Design review of the part shown in the three views and the two pictorial views. Dimensions are in mm from the part's minimum x, y and z. Give positions to 0.01 mm unless a question says otherwise; leave off trailing zeros. Loops run counter-clockwise (first coordinate to the right, second up) from the corner with the lowest first, then second, coordinate; pieces in that order, holes last.
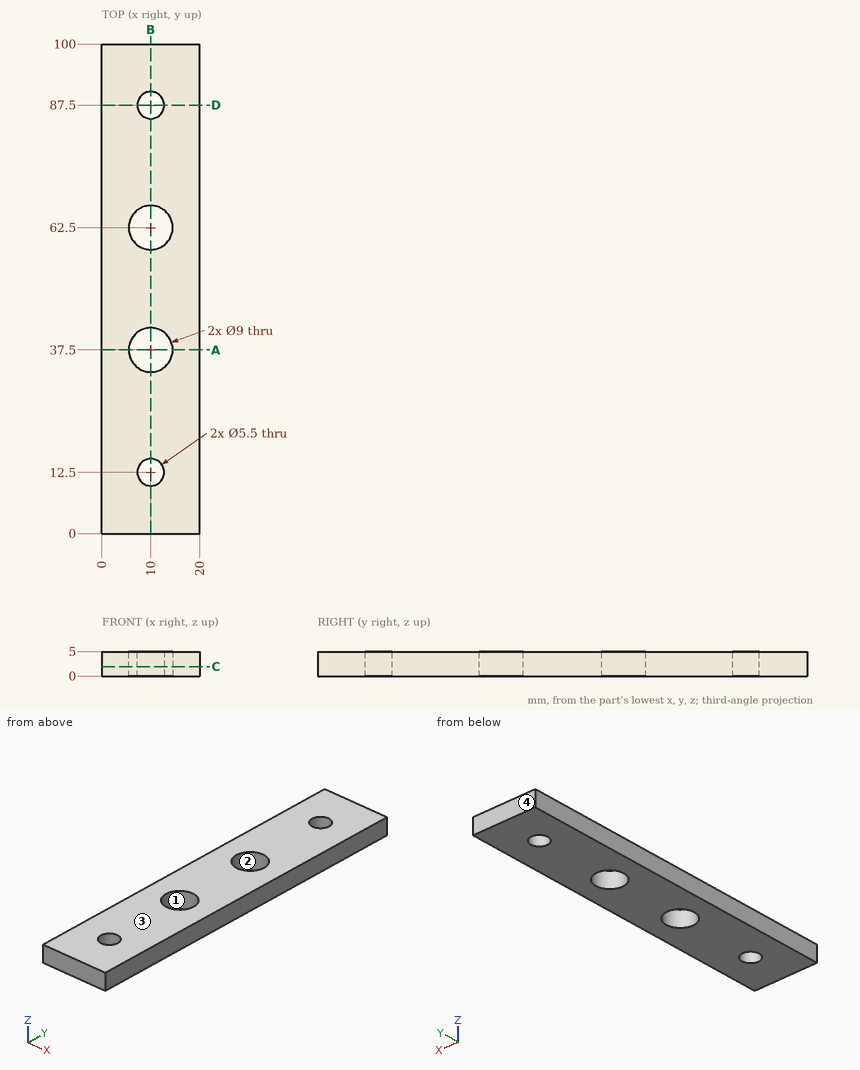
Q1. Consider section D-D on y = 87.5. Give the boundary of the cut face in (x, z).
Answers:
outline: (0, 0) - (7.25, 0) - (7.25, 5) - (0, 5) - close; (12.75, 0) - (20, 0) - (20, 5) - (12.75, 5) - close
Q2. For probe 1 along Y at (x, z) = (10, 3.35); probe 2 along Y at (x, z) = (8, 0.75); probe 3 along Y at (x, z) = (13.5, 2), list the stretches that pass through material, from the lowest coordinate up.
Answers:
probe 1: y = 0 to 9.75, 15.25 to 33, 42 to 58, 67 to 84.75, 90.25 to 100
probe 2: y = 0 to 10.61, 14.39 to 33.47, 41.53 to 58.47, 66.53 to 85.61, 89.39 to 100
probe 3: y = 0 to 34.67, 40.33 to 59.67, 65.33 to 100
Q3. Mouldability with a two-part tool opening along Y and no side actions: class the marked faces 1, 2, 3 and 4 as +Y half, -Y half, draft (parallel to the pull), parting line (faces both ways), or undercut.
Answers:
face 1: undercut
face 2: undercut
face 3: draft
face 4: +Y half
Q4. Consider section B-B on x = 10. Give the boundary of the cut face in (y, z).
Answers:
outline: (0, 0) - (9.75, 0) - (9.75, 5) - (0, 5) - close; (15.25, 0) - (33, 0) - (33, 5) - (15.25, 5) - close; (42, 0) - (58, 0) - (58, 5) - (42, 5) - close; (67, 0) - (84.75, 0) - (84.75, 5) - (67, 5) - close; (90.25, 0) - (100, 0) - (100, 5) - (90.25, 5) - close
Q5. Consider section A-A on y = 37.5. Give the boundary of the cut face in (x, z), plus the area to 3 significant figures.
Answers:
outline: (0, 0) - (5.5, 0) - (5.5, 5) - (0, 5) - close; (14.5, 0) - (20, 0) - (20, 5) - (14.5, 5) - close
area: 55.0 mm2
Q6. Consider section C-C on z = 1.9. Give the boundary of the cut face in (x, y).
Answers:
outline: (0, 0) - (20, 0) - (20, 100) - (0, 100) - close; hole circle Ø9 at (10, 37.5); hole circle Ø9 at (10, 62.5); hole circle Ø5.5 at (10, 12.5); hole circle Ø5.5 at (10, 87.5)
